Check sheet for the modelled part. Datum: model origin and axes. Units: mm. Face numbers are marked on the shaded views. A direction names the side the tool comes from. Coordinates: 2 decimals unless noted, no trailing zeros. Write each loop counter-clockwise with the first axis right and the second up, starting at its lowest first coordinate (ties: lowest second). Pieces come first, ordered by that corner, then holes. Notation, with made-up numbers: M 63.5,88.5 L 108.5,88.5 A24 ccw 108.5,113.5 Z; hole C -36,28 d10. An arc over 180 degrees is marked long. Answer as CSV lines item,"result". Start each with the question number.
1) Access from +Z, -Z, +X, -X, +Y, -Y to the whole of each face (thin tool, end or side, straight path). Record for the marked faces 1 and 2.
2) Material ranges on L1, parallel to X at y = 3.25, z = 3; L2, parallel to Z at x = 19, y = 0.25; L3, parallel to Z at x = 19, y = 2.75, recorded low to high. Write a range as [from, to].
3) Section check A-A (y = 0). Record the cut outline in (x, z).
4) Go/stop test with flat-tipped pins: pin 1 Ø5 at (x, z) = (13.5, -1) entering from -Y; pin 2 Ø1 at (y, z) = (-4, -4) entering from +X; pin 3 Ø5 at (x, y) = (1.5, -0.5) entering from +Z; pin 4 Ø1 at (x, y) = (6.5, -4) entering from +Z. Record where each tip stops, or that it passes through.
5) Section check C-C (x = 17.5). Record the cut outline in (y, z).
from build123d import *

# Parameters (mm, degrees)
SKETCH1_R           = 3
SHAFT_DEPTH         = 20
SKETCH2_R           = 6
BOSS_EXTRUDE2_DEPTH = 3
CHAMFER1_SIZE       = 0.25


with BuildPart() as part:
    # Sketch1 → SHAFT (new body)
    with BuildSketch(Plane(origin=(0, 0, 0), x_dir=(0, 0, -1), z_dir=(1, 0, 0))):
        Circle(SKETCH1_R)
    extrude(amount=SHAFT_DEPTH)

    # Sketch2 → Boss-Extrude2 (add)
    with BuildSketch(Plane.ZY):
        Circle(SKETCH2_R)
    extrude(amount=BOSS_EXTRUDE2_DEPTH)

    # Chamfer1
    chamfer1_edges = [part.edges().sort_by_distance(p)[0] for p in [
        (20, 0, 3),
        (0, 0, -6),
        (-3, 0, -6),
    ]]
    chamfer(chamfer1_edges, length=CHAMFER1_SIZE)


solid = part.part
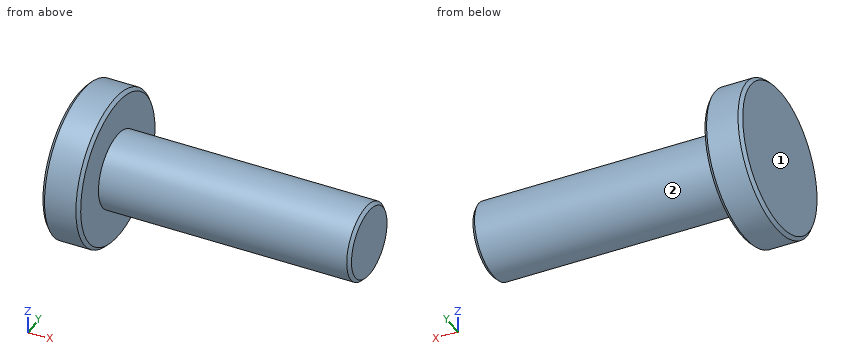
Results found:
1,face 1,"+Z, -Z, -X, +Y, -Y"
1,face 2,"+X"
2,L1,"x = [-3, 0]"
2,L2,"z = [-2.99, 2.99]"
2,L3,"z = [-1.2, 1.2]"
3,outline,"M -3,-5.75 L -2.75,-6 L -0.25,-6 L 0,-5.75 L 0,-3 L 19.75,-3 L 20,-2.75 L 20,2.75 L 19.75,3 L 0,3 L 0,5.75 L -0.25,6 L -2.75,6 L -3,5.75 Z"
4,pin 1,"stops at y = -3"
4,pin 2,"stops at x = 0"
4,pin 3,"stops at z = 6"
4,pin 4,"passes through"
5,outline,"C 0,0 d6"
